Verification items for the finished model (mm, model axes). Face numbers are marked on the shaded views. A direction names the side the tool comes from. Round coordinates to 2 decimals unless told otherwise and drop trailing zeros. Write each loop counter-clockwise with the first axis right and the second up, starting at its lowest first coordinate (ties: lowest second). Pieces come first, ordered by that corner, then holes. Notation, with made-up numbers: M -3.5,41 L 8.5,41 A12 ccw 8.5,60 Z; hole C 67,4 d11. An arc over 180 degrees is marked long. One line per item, written item: value. Start each with the question number.
Item 1: Gauge pin test, flat ends, axial feed: pin 1 (4.5 mm diameter, centred on x = 24, y = -61, fed in from +Z); pin 2 (12 mm diameter, centred on x = -22.5, y = -76, fed in from -Z); pin 3 (4 mm diameter, centred on x = -77.5, z = 52.5, fed in from +Y); pin 4 (6.5 mm diameter, centred on y = -54.2, z = 77.1, fed in from -X). Record the tip position at first contact, or that the pin passes through.
Item 2: Section check B-B, the plane y = -86.5. Record the cut outline in (x, z).
Item 3: Thickness scan on probe 1 along Z at (x, y) = (-49, -103.8); probe 2 along Y at (x, z) = (24, 48); probe 3 along X at (y, z) = (-103, 48.15). Record the ranges inside material, lowest first. Write a range as from..to.
Item 4: Draft check along X on the marked faces 6, 7, 8 and 9. Enter one of: +X half, -X half, draft (parallel to the pull), parting line (faces both ways), or undercut.
Item 5: Section check A-A, the plane z = 56.5. Record the cut outline in (x, y).
Item 6: Tool access check on the marked faces 1, 2, 3, 4 and 5. Record the directions out of +Z, -Z, +X, -X, +Y, -Y that give a thin tool (end or side, any length) a straight path to the whole face; none if there is none.
Item 7: Section check C-C, the plane z = 73. Record the cut outline in (x, y).
Item 8: Section check D-D, the plane y = -54.2. Record the cut outline in (x, z).
from build123d import *

# Parameters (mm, degrees)
CYLINDER382_R     = 2
CYLINDER382_DEPTH = 70
CYLINDER383_R     = 2
CYLINDER383_DEPTH = 70
BOX476_W          = 8.8
BOX476_H          = 52
BOX476_DEPTH      = 3
BOX473_W          = 41
BOX473_H          = 10
BOX473_DEPTH      = 3
BOX471_W          = 41
BOX471_H          = 9.9
BOX471_DEPTH      = 3
FILLET021_R       = 8
BOX411_W          = 6
BOX411_H          = 10
BOX411_DEPTH      = 16
BOX286_W          = 6
BOX286_H          = 9.9
BOX286_DEPTH      = 16
BOX409_W          = 6
BOX409_H          = 10
BOX409_DEPTH      = 16
BOX288_W          = 6
BOX288_H          = 20
BOX288_DEPTH      = 16
CYLINDER180_R     = 2
CYLINDER180_DEPTH = 33
CYLINDER179_R     = 2
CYLINDER179_DEPTH = 30
CYLINDER182_R     = 2
CYLINDER182_DEPTH = 33
CYLINDER181_R     = 2
CYLINDER181_DEPTH = 30
BOX408_W          = 20
BOX408_H          = 9
BOX408_DEPTH      = 20.1
BOX281_W          = 16
BOX281_H          = 9
BOX281_DEPTH      = 20.1
BOX283_W          = 66
BOX283_H          = 58.1
BOX283_DEPTH      = 3
CHAMFER044_SIZE   = 6.1
CYLINDER380_R     = 2
CYLINDER380_DEPTH = 65
CYLINDER381_R     = 2
CYLINDER381_DEPTH = 65
BOX475_W          = 8.8
BOX475_H          = 52
BOX475_DEPTH      = 3
BOX474_W          = 41
BOX474_H          = 10
BOX474_DEPTH      = 3
BOX472_W          = 41
BOX472_H          = 9.9
BOX472_DEPTH      = 3
FILLET019_R       = 8


with BuildPart() as cylinder382:
    # Cylinder382 → Cylinder382 (new body)
    with BuildSketch(Plane(origin=(-90, -103, -10), x_dir=(1, 0, 0), z_dir=(0, 0, 1))):
        Circle(CYLINDER382_R)
    extrude(amount=CYLINDER382_DEPTH)


with BuildPart() as fusion374:
    # Cylinder383 → Cylinder383 (new body)
    with BuildSketch(Plane(origin=(-90, -61, -10), x_dir=(1, 0, 0), z_dir=(0, 0, 1))):
        Circle(CYLINDER383_R)
    extrude(amount=CYLINDER383_DEPTH)

    # Fusion374: union Cylinder382
    add(cylinder382.part)


with BuildPart() as fusion374_1:
    # Fusion374 placement: moved
    add(fusion374.part.moved(Location((114, 0, 0))))


with BuildPart() as box476:
    # Box476 → Box476 (new body)
    with BuildSketch(Plane(origin=(25.2, -108, 46.1), x_dir=(1, 0, 0), z_dir=(0, 0, 1))):
        with Locations((4.4, 26)):
            Rectangle(BOX476_W, BOX476_H)
    extrude(amount=BOX476_DEPTH)


with BuildPart() as box473:
    # Box473 → Box473 (new body)
    with BuildSketch(Plane(origin=(-7, -66, 46.1), x_dir=(1, 0, 0), z_dir=(0, 0, 1))):
        with Locations((20.5, 5)):
            Rectangle(BOX473_W, BOX473_H)
    extrude(amount=BOX473_DEPTH)


with BuildPart() as fillet021:
    # Box471 → Box471 (new body)
    with BuildSketch(Plane(origin=(-7, -108, 46.1), x_dir=(1, 0, 0), z_dir=(0, 0, 1))):
        with Locations((20.5, 4.95)):
            Rectangle(BOX471_W, BOX471_H)
    extrude(amount=BOX471_DEPTH)

    # Fusion376: union Box476, Box473
    add(box476.part)
    add(box473.part)

    # Cut414: cut Fusion374
    add(fusion374_1.part, mode=Mode.SUBTRACT)

    # Fillet021
    fillet021_edges = [fillet021.edges().sort_by_distance(p)[0] for p in [
        (34, -108, 47.6),
        (34, -56, 47.6),
    ]]
    fillet(fillet021_edges, radius=FILLET021_R)


with BuildPart() as box411:
    # Box411 → Box411 (new body)
    with BuildSketch(Plane(origin=(-7, -66, 46.1), x_dir=(1, 0, 0), z_dir=(0, 0, 1))):
        with Locations((3, 5)):
            Rectangle(BOX411_W, BOX411_H)
    extrude(amount=BOX411_DEPTH)


with BuildPart() as box286:
    # Box286 → Box286 (new body)
    with BuildSketch(Plane(origin=(-67, -108, 46.1), x_dir=(1, 0, 0), z_dir=(0, 0, 1))):
        with Locations((3, 4.95)):
            Rectangle(BOX286_W, BOX286_H)
    extrude(amount=BOX286_DEPTH)


with BuildPart() as box409:
    # Box409 → Box409 (new body)
    with BuildSketch(Plane(origin=(-67, -66, 46.1), x_dir=(1, 0, 0), z_dir=(0, 0, 1))):
        with Locations((3, 5)):
            Rectangle(BOX409_W, BOX409_H)
    extrude(amount=BOX409_DEPTH)


with BuildPart() as fusion377:
    # Box288 → Box288 (new body)
    with BuildSketch(Plane(origin=(-7, -108, 46.1), x_dir=(1, 0, 0), z_dir=(0, 0, 1))):
        with Locations((3, 10)):
            Rectangle(BOX288_W, BOX288_H)
    extrude(amount=BOX288_DEPTH)

    # Fusion377: union Box411, Box286, Box409
    add(box411.part)
    add(box286.part)
    add(box409.part)


with BuildPart() as cylinder180:
    # Cylinder180 → Cylinder180 (new body)
    with BuildSketch(Plane(origin=(-74.6, -105.8, 63), x_dir=(0, 0, -1), z_dir=(1, 0, 0))):
        Circle(CYLINDER180_R)
    extrude(amount=CYLINDER180_DEPTH)


with BuildPart() as fusion247:
    # Cylinder179 → Cylinder179 (new body)
    with BuildSketch(Plane(origin=(-71.6, -105.8, 73), x_dir=(0, 0, -1), z_dir=(1, 0, 0))):
        Circle(CYLINDER179_R)
    extrude(amount=CYLINDER179_DEPTH)

    # Fusion247: union Cylinder180
    add(cylinder180.part)


with BuildPart() as fusion247_1:
    # Fusion247 placement: moved
    add(fusion247.part.moved(Location((0, 2, 4))))


with BuildPart() as cylinder182:
    # Cylinder182 → Cylinder182 (new body)
    with BuildSketch(Plane(origin=(-74.6, -56.2, 63), x_dir=(0, 0, -1), z_dir=(1, 0, 0))):
        Circle(CYLINDER182_R)
    extrude(amount=CYLINDER182_DEPTH)


with BuildPart() as fusion252:
    # Cylinder181 → Cylinder181 (new body)
    with BuildSketch(Plane(origin=(-71.6, -56.2, 73), x_dir=(0, 0, -1), z_dir=(1, 0, 0))):
        Circle(CYLINDER181_R)
    extrude(amount=CYLINDER181_DEPTH)

    # Fusion246: union Cylinder182
    add(cylinder182.part)


with BuildPart() as fusion252_1:
    # Fusion246 placement: moved
    add(fusion252.part.moved(Location((0, 2, 4))))

    # Fusion252: union Fusion247
    add(fusion247_1.part)


with BuildPart() as box408:
    # Box408 → Box408 (new body)
    with BuildSketch(Plane(origin=(-64.3, -58.9, 62), x_dir=(1, 0, 0), z_dir=(0, 0, 1))):
        with Locations((10, 4.5)):
            Rectangle(BOX408_W, BOX408_H)
    extrude(amount=BOX408_DEPTH)


with BuildPart() as box281:
    # Box281 → Box281 (new body)
    with BuildSketch(Plane(origin=(-60.3, -108, 62), x_dir=(1, 0, 0), z_dir=(0, 0, 1))):
        with Locations((8, 4.5)):
            Rectangle(BOX281_W, BOX281_H)
    extrude(amount=BOX281_DEPTH)


with BuildPart() as chamfer044:
    # Box283 → Box283 (new body)
    with BuildSketch(Plane(origin=(-71.6, -108, 59), x_dir=(1, 0, 0), z_dir=(0, 0, 1))):
        with Locations((33, 29.05)):
            Rectangle(BOX283_W, BOX283_H)
    extrude(amount=BOX283_DEPTH)

    # Fusion372: union Box408, Box281
    add(box408.part)
    add(box281.part)

    # Cut412: cut Fusion252
    add(fusion252_1.part, mode=Mode.SUBTRACT)


with BuildPart() as chamfer044_1:
    # Cut412 placement: moved
    add(chamfer044.part.moved(Location((4.7, 0, 0.1))))

    # Chamfer044
    chamfer044_edges = [chamfer044_1.edges().sort_by_distance(p)[0] for p in [
        (-66.9, -49.9, 60.6),
        (-0.9, -49.9, 60.6),
    ]]
    chamfer(chamfer044_edges, length=CHAMFER044_SIZE)


with BuildPart() as chamfer044_2:
    # Chamfer044 placement: moved
    add(chamfer044_1.part.moved(Location((-0.1, 0, 0))))


with BuildPart() as cylinder380:
    # Cylinder380 → Cylinder380 (new body)
    with BuildSketch(Plane(origin=(-90, -103, -10), x_dir=(1, 0, 0), z_dir=(0, 0, 1))):
        Circle(CYLINDER380_R)
    extrude(amount=CYLINDER380_DEPTH)


with BuildPart() as fusion373:
    # Cylinder381 → Cylinder381 (new body)
    with BuildSketch(Plane(origin=(-90, -61, -10), x_dir=(1, 0, 0), z_dir=(0, 0, 1))):
        Circle(CYLINDER381_R)
    extrude(amount=CYLINDER381_DEPTH)

    # Fusion373: union Cylinder380
    add(cylinder380.part)


with BuildPart() as fusion373_1:
    # Fusion373 placement: moved
    add(fusion373.part.moved(Location((-2, 0, 0))))


with BuildPart() as box475:
    # Box475 → Box475 (new body)
    with BuildSketch(Plane(origin=(-102, -108, 46.1), x_dir=(1, 0, 0), z_dir=(0, 0, 1))):
        with Locations((4.4, 26)):
            Rectangle(BOX475_W, BOX475_H)
    extrude(amount=BOX475_DEPTH)


with BuildPart() as box474:
    # Box474 → Box474 (new body)
    with BuildSketch(Plane(origin=(-102, -66, 46.1), x_dir=(1, 0, 0), z_dir=(0, 0, 1))):
        with Locations((20.5, 5)):
            Rectangle(BOX474_W, BOX474_H)
    extrude(amount=BOX474_DEPTH)


with BuildPart() as rescue_arm_stand:
    # Box472 → Box472 (new body)
    with BuildSketch(Plane(origin=(-102, -108, 46.1), x_dir=(1, 0, 0), z_dir=(0, 0, 1))):
        with Locations((20.5, 4.95)):
            Rectangle(BOX472_W, BOX472_H)
    extrude(amount=BOX472_DEPTH)

    # Fusion375: union Box475, Box474
    add(box475.part)
    add(box474.part)

    # Cut413: cut Fusion373
    add(fusion373_1.part, mode=Mode.SUBTRACT)

    # Fillet019
    fillet019_edges = [rescue_arm_stand.edges().sort_by_distance(p)[0] for p in [
        (-102, -108, 47.6),
        (-102, -56, 47.6),
    ]]
    fillet(fillet019_edges, radius=FILLET019_R)

    # Fusion378: union Fillet021, Fusion377, Chamfer044
    add(fillet021.part)
    add(fusion377.part)
    add(chamfer044_2.part)


solid = rescue_arm_stand.part
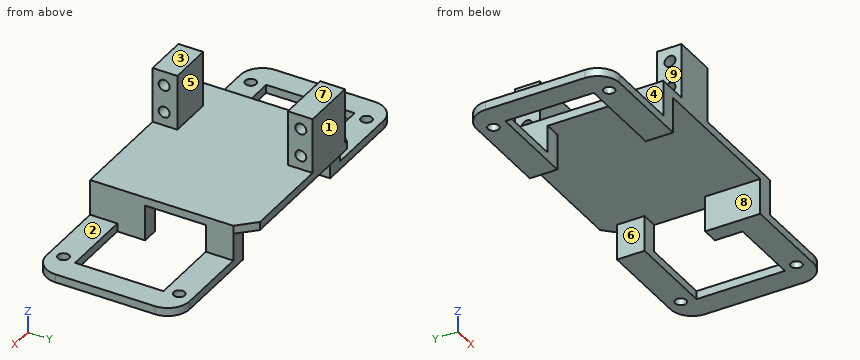
Response values:
1. pin 1: stops at z = 49.1
1. pin 2: stops at z = 59.1
1. pin 3: passes through
1. pin 4: stops at x = -59.7
2. outline: M -102,46.1 L -93.2,46.1 L -93.2,49.1 L -102,49.1 Z; M -67,59.1 L -1,59.1 L -1,62.1 L -67,62.1 Z; M 25.2,46.1 L 34,46.1 L 34,49.1 L 25.2,49.1 Z
3. probe 1: z = 59.1..65.1, 69.1..75.1, 79.1..82.2
3. probe 2: y = -108..-105, -101..-98.1, -66..-63, -59..-56
3. probe 3: x = -101.42..-94, -90..-61, -7..22, 26..33.42
4. face 6: undercut
4. face 7: draft
4. face 8: undercut
4. face 9: -X half
5. outline: M -67,-108 L -61,-108 L -61,-98.1 L -67,-98.1 Z; M -67,-66 L -61,-66 L -61,-56 L -67,-56 Z; M -7,-108 L -1,-108 L -1,-88 L -7,-88 Z; M -7,-66 L -1,-66 L -1,-56 L -7,-56 Z
6. face 1: +Z, -Z, +X, -X, +Y
6. face 2: +Z, +X, +Y, -Y
6. face 3: +Z, +X, -X, +Y, -Y
6. face 4: +Z, -X, +Y, -Y
6. face 5: +Z, +X, -X
7. outline: M -59.7,-58.9 L -39.7,-58.9 L -39.7,-49.9 L -59.7,-49.9 Z; M -55.7,-108 L -39.7,-108 L -39.7,-99 L -55.7,-99 Z
8. outline: M -65.2,59.1 L -2.8,59.1 L -2.8,62.1 L -39.7,62.1 L -39.7,65.1 L -59.7,65.1 L -59.7,62.1 L -65.2,62.1 Z; M -59.7,69.1 L -39.7,69.1 L -39.7,75.1 L -59.7,75.1 Z; M -59.7,79.1 L -39.7,79.1 L -39.7,82.2 L -59.7,82.2 Z
